The listing builds one solid part. Answer for the finished solid, in the listing's coordinates (mm). A direction names the side the tool comes from. Coordinates: 2 decimals unless noted, no trailing zeros. Loops run counter-clockwise (first coordinate to the right, second up) from the corner with the lowest first, then second, coordinate; pieces in that order, holes last. Notation, with made-up numbers: (-25.75, 7) - (23.25, 7) arc R37 ccw to (23.25, 44) - close; hole circle Ø7 at (80, 87). An arc over 180 degrees is marked (long way). Return JSON: item names as keys, results as strings. Group by question number.
1. Section A-A (y = 0) is taken. Write down the section's boundary in (x, z).
2. This flat-tipped pin is pushed along its axis until it touches: P1, Ø10, axis at y = -1.5, z = 1, coming from the -X side. Where does it stop, or does it pass through?
3. Section B-B (z = 0) is taken. Write down the section's boundary in (x, y), and give its area (3 significant figures).
4. Find the intervals of material crossed by line 1 along X through (y, z) = (-2, 10.25); line 2 along Y through (x, z) = (-1.5, 3.75); line 3 along Y through (x, z) = (-3.65, 0), in increasing order.
5. Section D-D (z = -13) is taken. Write down the section's boundary in (x, y).
6. The mould has two halves that part along Z. Classify faces 3 (the face through (2.5, -9, 4)), 4 (the face through (-3, 0, -15)), 5 (the face through (-3.732, 2.867, -9.104)): pulls with the +Z half, pulls with the -Z half, needs draft (parallel to the pull), parting line crosses it, or undercut.
7. Section C-C (x = 0) is taken. Write down the section's boundary in (y, z).
8. Which of the six approach directions +Z, -Z, +X, -X, +Y, -Y give full straight-line access (tool end or side, diameter ignored) to faces 1 (the face through (-2.5, -9, 4)), 2 (the face through (3.768, 2.867, -9.104))?
```python
from build123d import *

# Parameters (mm, degrees)
SKETCH_1_W          = 10
SKETCH_1_H          = 30
SKETCH_1_W_2        = 5
SKETCH_1_H_2        = 20
EXTRUDE_1_DEPTH     = 15
SKETCH_2_R          = 9.544400842
CUT_EXTRUDE_1_DEPTH = 30


with BuildPart() as part:
    # 草图1 → 凸台-拉伸1 (new, symmetric)
    with BuildSketch(Plane.XY):
        Rectangle(SKETCH_1_W, SKETCH_1_H)
        Rectangle(SKETCH_1_W_2, SKETCH_1_H_2, mode=Mode.SUBTRACT)
    extrude(amount=EXTRUDE_1_DEPTH, both=True)

    # 草图2 → 切除-拉伸1 (cut)
    with BuildSketch(Plane(origin=(5, 0, 0), x_dir=(0, 0, -1), z_dir=(1, 0, 0))):
        Circle(SKETCH_2_R)
    extrude(amount=-CUT_EXTRUDE_1_DEPTH, mode=Mode.SUBTRACT)


solid = part.part
```
The answers:
{
 "1": {"outline": "(-5, -15) - (-2.5, -15) - (-2.5, -9.54) - (-5, -9.54) - close; (-5, 9.54) - (-2.5, 9.54) - (-2.5, 15) - (-5, 15) - close; (2.5, -15) - (5, -15) - (5, -9.54) - (2.5, -9.54) - close; (2.5, 9.54) - (5, 9.54) - (5, 15) - (2.5, 15) - close"},
 "2": {"P1": "passes through"},
 "3": {"outline": "(-5, -15) - (5, -15) - (5, -9.54) - (2.5, -9.54) - (2.5, -10) - (-2.5, -10) - (-2.5, -9.54) - (-5, -9.54) - close; (-5, 9.54) - (-2.5, 9.54) - (-2.5, 10) - (2.5, 10) - (2.5, 9.54) - (5, 9.54) - (5, 15) - (-5, 15) - close", "area": "105 mm2"},
 "4": {"line 1": "x = -5 to -2.5, 2.5 to 5", "line 2": "y = -15 to -10, 10 to 15", "line 3": "y = -15 to -9.54, 9.54 to 15"},
 "5": {"outline": "(-5, -15) - (5, -15) - (5, 15) - (-5, 15) - close; hole (-2.5, -10) - (2.5, -10) - (2.5, 10) - (-2.5, 10) - close"},
 "6": {"face 3": "needs draft", "face 4": "pulls with the -Z half", "face 5": "undercut"},
 "7": {"outline": "(-15, -15) - (-10, -15) - (-10, 15) - (-15, 15) - close; (10, -15) - (15, -15) - (15, 15) - (10, 15) - close"},
 "8": {"face 1": "+Z, -Z", "face 2": "+X, -X"}
}
